The model under review builds one solid part; all positions refer to its coordinate system, in mm. Face numbers are marked on the shaded views. A direction names the side the tool comes from. Give positions to 0.01 mm unless a question says otherwise; leave off trailing zeros. Loops run counter-clockwise (first coordinate to the right, second up) from the corner with the lowest first, then second, coordinate; pieces in that order, holes last. Notation, with made-up numbers: (69, -19) -> (106, -19) arc R19 ccw to (106, -7) -> close; hole circle Ø2 at (-8.5, 46). An arc over 180 degrees is marked (long way). Write each question's results on one line, items separated by ' | '. Start each with the question number.
Q1. We need section B-B (x = -16.5). Write out the cut boundary in (y, z), plus the area to 3 significant figures.
Q2. We need section D-D (x = -6). Write out the cut boundary in (y, z), plus the area to 3 significant figures.
Q3. Machinability: for the marked faces 1, 2 and 3, which of the approach directions +Z, -Z, +X, -X, +Y, -Y give a long, thin tool a straight path to every point of the face, cutting with its end or side? Answer none if there is none.
Q4. We need section C-C (y = -0.5). Write out the cut boundary in (x, z), plus the area to 3 significant figures.
Q5. Mouldability with a two-part tool opening along Y and no side actions: class the marked faces 4, 5, 6 and 7 as released by +Y, released by -Y, zero draft, split by the parting line, or undercut.
Q6. Insertion check: pin 1 Ø0.6 at (y, z) = (0, 8) entering from -X; pin 2 Ø4.5 at (x, y) = (21.5, -0.5) entering from +Z; pin 3 Ø0.6 at (y, z) = (0, 8.5) entering from +X. Each pin has a flat end and moves straight along its axis. Give the tip position at first contact, or say it passes through.
Q7. Wall thickness on L1, parallel to Y at x = 21.5, z = 8; L2, parallel to X at y = 1.75, z = 9.75; L3, parallel to Z at x = -11, y = -0.5: over which ranges is each line inside the solid? List them lowest first. Write a range as [from, to].
Q8. We need section A-A (z = 7). Write out the cut boundary in (x, y).
from build123d import *

# Parameters (mm, degrees)
F0_W     = 55
F0_H     = 15.6
F1_DEPTH = 11
F2_W     = 2
F2_H     = 2
F3_DEPTH = 5
F4_W     = 19
F4_H     = 9.6
F5_DEPTH = 9
F6_R     = 2
F7_SIZE  = 0.2
F8_SIZE  = 0.8


with BuildPart() as f1:
    # F0 (on Top) → F1 (new body)
    with BuildSketch(Plane.XY):
        Rectangle(F0_W, F0_H)
    extrude(amount=F1_DEPTH)

    # F2 (on face) → F3 (cut)
    with BuildSketch(Plane.XY.offset(11)):
        with Locations((-5.77, 0)):
            Rectangle(F2_W, F2_H)
    extrude(amount=-F3_DEPTH, mode=Mode.SUBTRACT)

    # F4 (on face) → F5 (cut)
    with BuildSketch(Plane.XY.offset(11)):
        with Locations((-18, 0)):
            Rectangle(F4_W, F4_H)
        with Locations((18, 0)):
            Rectangle(F4_W, F4_H)
    extrude(amount=-F5_DEPTH, mode=Mode.SUBTRACT)

    # F6
    f6_edges = [f1.edges().sort_by_distance(p)[0] for p in [
        (-8.5, 4.8, 6.5),
        (-18, 4.8, 2),
        (-8.5, 0, 2),
        (-18, -4.8, 2),
        (-8.5, -4.8, 6.5),
        (8.5, 0, 2),
        (8.5, 4.8, 6.5),
        (18, 4.8, 2),
        (18, -4.8, 2),
        (8.5, -4.8, 6.5),
    ]]
    fillet(f6_edges, radius=F6_R)

    # F7
    f7_edges = [f1.edges().sort_by_distance(p)[0] for p in [
        (-19, -4.8, 11),
        (-9.085786, -4.214214, 11),
        (-27.5, -6.3, 11),
        (-8.5, 0, 11),
        (0, -7.8, 11),
        (-9.085786, 4.214214, 11),
        (27.5, -6.3, 11),
        (-19, 4.8, 11),
        (19, -4.8, 11),
        (-27.5, 6.3, 11),
        (9.085786, -4.214214, 11),
        (0, 7.8, 11),
        (8.5, 0, 11),
        (27.5, 6.3, 11),
        (9.085786, 4.214214, 11),
        (19, 4.8, 11),
        (-6.77, 0, 11),
        (-5.77, 1, 11),
        (-5.77, -1, 11),
        (-4.77, 0, 11),
    ]]
    chamfer(f7_edges, length=F7_SIZE)

    # F8
    f8_edges = [f1.edges().sort_by_distance(p)[0] for p in [
        (27.5, 0, 0),
        (0, 7.8, 0),
        (-27.5, 0, 0),
        (0, -7.8, 0),
    ]]
    chamfer(f8_edges, length=F8_SIZE)


solid = f1.part
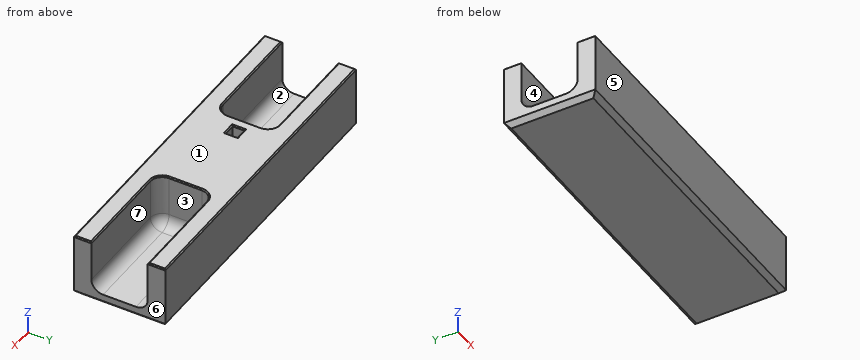
Output:
1) outline: (-7.8, 0.8) -> (-7, 0) -> (7, 0) -> (7.8, 0.8) -> (7.8, 10.8) -> (7.6, 11) -> (5, 11) -> (4.8, 10.8) -> (4.8, 4) arc R2 cw to (2.8, 2) -> (-2.8, 2) arc R2 cw to (-4.8, 4) -> (-4.8, 10.8) -> (-5, 11) -> (-7.6, 11) -> (-7.8, 10.8) -> close | area: 86.2 mm2
2) outline: (-7.8, 0.8) -> (-7, 0) -> (7, 0) -> (7.8, 0.8) -> (7.8, 10.8) -> (7.6, 11) -> (1.2, 11) -> (1, 10.8) -> (1, 6) -> (-1, 6) -> (-1, 10.8) -> (-1.2, 11) -> (-7.6, 11) -> (-7.8, 10.8) -> close | area: 161 mm2
3) face 1: +Z, +X, -X, +Y, -Y | face 2: +Z, -X | face 3: +Z, +X
4) outline: (-27.5, 0.8) -> (-26.7, 0) -> (26.7, 0) -> (27.5, 0.8) -> (27.5, 2) -> (10.5, 2) arc R2 cw to (8.5, 4) -> (8.5, 10.8) -> (8.3, 11) -> (-4.57, 11) -> (-4.77, 10.8) -> (-4.77, 6) -> (-6.77, 6) -> (-6.77, 10.8) -> (-6.97, 11) -> (-8.3, 11) -> (-8.5, 10.8) -> (-8.5, 4) arc R2 cw to (-10.5, 2) -> (-27.5, 2) -> close | area: 254 mm2
5) face 4: undercut | face 5: released by -Y | face 6: zero draft | face 7: undercut
6) pin 1: x = -8.5 | pin 2: z = 2 | pin 3: x = 8.5
7) L1: [-7.8, -4.8], [4.8, 7.8] | L2: [-8.5, 8.5] | L3: [0, 2]
8) outline: (-27.5, -7.8) -> (27.5, -7.8) -> (27.5, -4.8) -> (10.5, -4.8) arc R2 cw to (8.5, -2.8) -> (8.5, 2.8) arc R2 cw to (10.5, 4.8) -> (27.5, 4.8) -> (27.5, 7.8) -> (-27.5, 7.8) -> (-27.5, 4.8) -> (-10.5, 4.8) arc R2 cw to (-8.5, 2.8) -> (-8.5, -2.8) arc R2 cw to (-10.5, -4.8) -> (-27.5, -4.8) -> close; hole (-6.77, -1) -> (-4.77, -1) -> (-4.77, 1) -> (-6.77, 1) -> close
